The listing builds one solid part. Answer for the finished solid, in the listing's coordinates (mm). Give positions to 0.01 mm unless a question says otherwise; leave off trailing zeros. Write each loop counter-clockwise with the first axis right and the second up, starting at its lowest first coordinate (ties: lowest second). Pieces come first, ordered by that corner, then holes. Notation, with made-up numbers: (58.5, 81) -> (110.5, 81) arc R24 ccw to (110.5, 109) -> close; hole circle Ø4 at (-2, 3.25). An arc over 180 degrees is marked (long way). One line per question, with ' | ' between items.
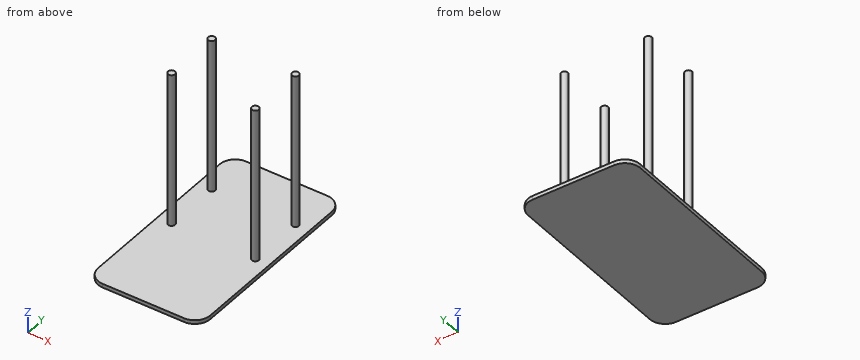
from build123d import *

# Parameters (mm, degrees)
F0_R     = 1.143
F1_DEPTH = 50.8
F2_DEPTH = 1.27


with BuildPart() as f1:
    # F0 (on Top) → F1 (new body)
    with BuildSketch(Plane.XY):
        with Locations((-13.479616519, -10.2275963136)):
            Circle(F0_R)
    extrude(amount=F1_DEPTH)



with BuildPart() as f1b:
    # F0 (on Top) → F1, piece 2 (new body)
    with BuildSketch(Plane.XY):
        with Locations((-13.479616519, 8.5684026553)):
            Circle(F0_R)
    extrude(amount=F1_DEPTH)


with BuildPart() as f1c:
    # F0 (on Top) → F1, piece 3 (new body)
    with BuildSketch(Plane.XY):
        with Locations((14.1555836841, 8.5684026553)):
            Circle(F0_R)
    extrude(amount=F1_DEPTH)


with BuildPart() as f1d:
    # F0 (on Top) → F1, piece 4 (new body)
    with BuildSketch(Plane.XY):
        with Locations((14.1555836841, -10.2275963136)):
            Circle(F0_R)
    extrude(amount=F1_DEPTH)


with BuildPart() as f1_1:
    add(f1.part)

    add(f1b.part)  # F2 merges F1b

    add(f1c.part)  # F2 merges F1c

    add(f1d.part)  # F2 merges F1d
    # F0 (on Top) → F2 (join)
    with BuildSketch(Plane.XY):
        with BuildLine():
            ThreePointArc((18.8266877085, 18.9855317903), (17.3387901569, 22.5776342387), (13.7466877085, 24.0655317903))
            Line((13.7466877085, 24.0655317903), (-13.0707205434, 24.0655317903))
            ThreePointArc((-13.0707205434, 24.0655317903), (-16.6628229918, 22.5776342387), (-18.1507205434, 18.9855317903))
            Line((-18.1507205434, 18.9855317903), (-18.1507205434, -20.6447254485))
            Line((-18.1507205434, -20.6447254485), (-18.1507205434, -38.0270736456))
            ThreePointArc((-18.1507205434, -38.0270736456), (-16.6628229918, -41.619176094), (-13.0707205434, -43.1070736456))
            Line((-13.0707205434, -43.1070736456), (13.7466877085, -43.1070736456))
            ThreePointArc((13.7466877085, -43.1070736456), (17.3387901569, -41.619176094), (18.8266877085, -38.0270736456))
            Line((18.8266877085, -38.0270736456), (18.8266877085, -20.6447254485))
            Line((18.8266877085, -20.6447254485), (18.8266877085, 18.9855317903))
        make_face()
        with Locations((-13.479616519, -10.2275963136)):
            Circle(F0_R, mode=Mode.SUBTRACT)
        with Locations((14.1555836841, -10.2275963136)):
            Circle(F0_R, mode=Mode.SUBTRACT)
        with Locations((-13.479616519, 8.5684026553)):
            Circle(F0_R, mode=Mode.SUBTRACT)
        with Locations((14.1555836841, 8.5684026553)):
            Circle(F0_R, mode=Mode.SUBTRACT)
        with Locations((14.1555836841, -10.2275963136)):
            Circle(F0_R)
        with Locations((-13.479616519, -10.2275963136)):
            Circle(F0_R)
        with Locations((-13.479616519, 8.5684026553)):
            Circle(F0_R)
        with Locations((14.1555836841, 8.5684026553)):
            Circle(F0_R)
    extrude(amount=-F2_DEPTH)


solid = f1_1.part
Item 1: Find section C-C (x = -9). Write down the section's boundary in (y, z), then the cut area to 3 significant figures.
Answers below:
outline: (-43.11, -1.27) -> (24.07, -1.27) -> (24.07, 0) -> (-43.11, 0) -> close | area: 85.3 mm²
Item 2: Find section B-B (z = 36). Write down the section's boundary in (x, y), then the cut area to 3 significant figures.
Answers below:
outline: circle Ø2.29 at (-13.48, -10.23); circle Ø2.29 at (-13.48, 8.57); circle Ø2.29 at (14.16, -10.23); circle Ø2.29 at (14.16, 8.57) | area: 16.4 mm²
Item 3: Flat-ended cylindrical pins translate along their axes: pin 1 (8 mm diameter, centred on x = -3.5, y = 14, fed in from +Z); pin 2 (8 mm diameter, centred on x = 12.5, z = 15.5, fed in from -Y); pin 3 (8 mm diameter, centred on y = -15, z = 45, fed in from -X). Find the tip coordinate at first contact, or state that the pin passes through.
Answers below:
pin 1: z = 0 | pin 2: y = -11.37 | pin 3: x = -14.32
Item 4: Find section A-A (y = -19). Write down the section's boundary in (x, z), then the cut area to 3 significant figures.
Answers below:
outline: (-18.15, -1.27) -> (18.83, -1.27) -> (18.83, 0) -> (-18.15, 0) -> close | area: 47.0 mm²
Item 5: Consider line 1 (Z direction, x = -8, y = -31.5). Determine where the line is inside the solid, lowest interval first. Write a range as [from, to].
Answers below:
line 1: [-1.27, 0]
